```python
from build123d import *

# Parameters (mm, degrees)
F0_R        = 2
F1_DEPTH    = 4
F3_DEPTH    = 20
F5_DEPTH    = 20
F6_T1_DEPTH = 10.5320888862
F6_T3_DEPTH = 10.5320888862
F7_R        = 0.5
F8_R        = 0.25
F9_DEPTH    = 3


# Not quite as in the source:
# - a fillet or chamfer that OpenCascade refuses, or shapes differently, is made with other operations: its cross-section is extruded or revolved along the edge and cut away or added


with BuildPart() as f1:
    # F0 (on Top) → F1 (new body)
    with BuildSketch(Plane.XY):
        Circle(F0_R)
    extrude(amount=F1_DEPTH)

    # F2 (on Right) → F3 (join)
    with BuildSketch(Plane.YZ):
        Polygon((2, 3.0320888862), (-2, 1.5762079492), (-2, 1.0441190629), (2, 2.5), align=None)
    extrude(amount=F3_DEPTH)

    # F4 (on Right) → F5 (join)
    with BuildSketch(Plane.YZ):
        Polygon((2, 1.0441190629), (2, 1.5762079492), (-2, 3.0320888862), (-2, 2.5), align=None)
    extrude(amount=-F5_DEPTH)

    # F6: fillet of radius 2 on 4 edges, made by hand

    # F6_s2 → F6_t1 (cut)
    with BuildSketch(Plane.XY.offset(-3.9558809371)):
        with BuildLine():
            ThreePointArc((-18, 2), (-19.4142135624, 1.4142135624), (-20, 0))
            Line((-20, 0), (-20, 2))
            Line((-20, 2), (-18, 2))
        make_face()
        with BuildLine():
            ThreePointArc((18, -2), (19.4142135624, -1.4142135624), (20, 0))
            Line((20, 0), (20, -2))
            Line((20, -2), (18, -2))
        make_face()
    extrude(amount=F6_T1_DEPTH, mode=Mode.SUBTRACT)

    # F6_s4 → F6_t3 (cut)
    with BuildSketch(Plane.XY.offset(-2.5)):
        with BuildLine():
            ThreePointArc((-18, -2), (-19.4142135624, -1.4142135624), (-20, 0))
            Line((-20, 0), (-20, -2))
            Line((-20, -2), (-18, -2))
        make_face()
        with BuildLine():
            ThreePointArc((18, 2), (19.4142135624, 1.4142135624), (20, 0))
            Line((20, 0), (20, 2))
            Line((20, 2), (18, 2))
        make_face()
    extrude(amount=F6_T3_DEPTH, mode=Mode.SUBTRACT)

    # F7
    f7_edges = [f1.edges().sort_by_distance(p)[0] for p in [
        (-2, 0, 4),
    ]]
    fillet(f7_edges, radius=F7_R)

    # F8 (on face) → F9 (cut)
    with BuildSketch(Plane(origin=(0, 0, 0), x_dir=(1, 0, 0), z_dir=(0, 0, -1))):
        Circle(F8_R)
    extrude(amount=-F9_DEPTH, mode=Mode.SUBTRACT)


solid = f1.part
```
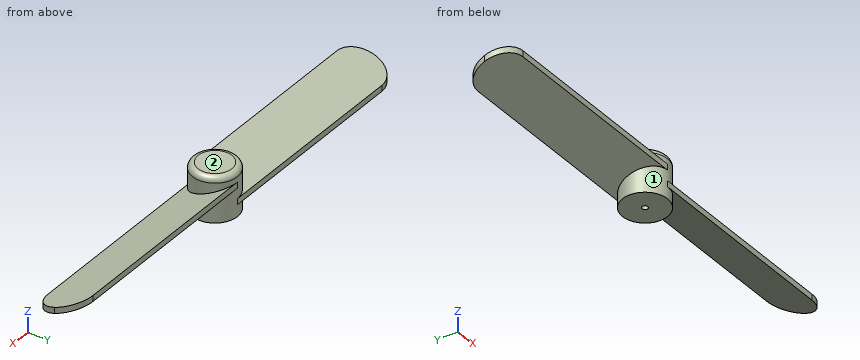
Can you work these out from the model? Positions are in its coordinate system, mm. Face numbers are marked on the shaded views. A direction names the side the tool comes from. Round coordinates to 2 decimals unless told otherwise and drop trailing zeros. Loops run counter-clockwise (first coordinate to the right, second up) from the corner with the lowest first, then second, coordinate; pieces in that order, holes last.
Item 1: Will this pin go through, and if not, where does the flat tip stop? pin 1 Ø1.5 at (x, y) = (9, 0.5) entering from -Z.
Item 2: Please list where these lines run through material, in increasing order: L1, parallel to Y at x = 0, z = 2.4; L2, parallel to Z at x = -17.5, y = 0.15.
Item 3: Suppose I cut it at A-A, the plane x = 11. Write out the boundary of the cut face in (y, z), then the cut area to 3 significant figures.
Item 4: Which directions (+Z, -Z, +X, -X, +Y, -Y) give clear straight access to the entire face, cutting with the end or side of a thin tool? Please do the marked faces 1 and 2.
Reported:
1. pin 1: stops at z = 1.68
2. L1: y = -2 to -0.25, 0.25 to 2
2. L2: z = 1.72 to 2.25
3. outline: (-2, 1.04) - (2, 2.5) - (2, 3.03) - (-2, 1.58) - close
3. area: 2.13 mm2
4. face 1: none
4. face 2: +Z, +X, -X, +Y, -Y
